```python
from build123d import *

# Parameters (mm, degrees)
BOSS_EXTRUDE1_START             = -14.3
SKETCH1_W                       = 40
SKETCH1_H                       = 55
BOSS_EXTRUDE1_DEPTH             = 31.35
F_7_64_0_10938_DIAMETER_HOLE1_D = 2.778252


with BuildPart() as part:
    # Sketch1 → Boss-Extrude1 (new body)
    with BuildSketch(Plane(origin=(0, 205.794413587, 0), x_dir=(1, 0, 0), z_dir=(0, 1, 0)).offset(BOSS_EXTRUDE1_START)):
        with Locations((59.936494412, -210.044134902)):
            Rectangle(SKETCH1_W, SKETCH1_H)
    extrude(amount=BOSS_EXTRUDE1_DEPTH)

    # 7/64 (0.10938) Diameter Hole1 (through all)
    with Locations(Plane(origin=(0, 191.494413587, 0), x_dir=(-1, 0, 0), z_dir=(0, -1, 0))):
        with Locations((-75.836494412, -186.444134902), (-43.836494412, -233.444134902)):
            Hole(F_7_64_0_10938_DIAMETER_HOLE1_D / 2)


solid = part.part
```
The model under review builds one solid part; all positions refer to its coordinate system, in mm. Give positions to 0.01 mm unless a question says otherwise; leave off trailing zeros. Write each question's results on one line, items separated by ' | '. Start each with the question number.
1. Insertion check: pin 1 Ø4.5 at (x, z) = (75.84, 186.44) entering from +Y; pin 2 Ø2.5 at (x, z) = (43.84, 233.44) entering from +Y. Each pin has a flat end and moves straight along its axis. Give the tip position at first contact, or say it passes through.
2. Mouldability with a two-part tool opening along X and no side actions: class faces 1 (the cylindrical face through (76.477, 207.389, 187.677)), 2 (the flat face through (60, 207, 237.544)), 3 (the flat face through (79.936, 207, 210)) as released by +X, released by -X, zero draft, split by the parting line, or undercut.
3. For probe 1 along Z at (x, y) = (75.5, 200.5); probe 2 along Z at (x, y) = (77, 211.5); probe 3 along X at (y, z) = (216.5, 234.5), list the stretches that pass through material, from the lowest coordinate up. Write a range as [from, to].
Results found:
1) pin 1: stops at y = 222.84 | pin 2: passes through
2) face 1: undercut | face 2: zero draft | face 3: released by +X
3) probe 1: z = [182.54, 185.1], [187.79, 237.54] | probe 2: z = [182.54, 185.69], [187.2, 237.54] | probe 3: x = [39.94, 42.93], [44.74, 79.94]
